from build123d import *

# Parameters (mm, degrees)
SKETCH_3_R               = 3
EXTRUDE_6_DEPTH          = 0.001
EXTRUDE_6_2_DEPTH        = 0.001
EXTRUDE_6_3_DEPTH        = 0.001
EXTRUDE_6_4_DEPTH        = 0.001
SKETCH_11_R              = 2.25
CUT_EXTRUDE_2_DEPTH      = 1
CUT_EXTRUDE_2_DEPTH_BACK = 1.001
EXTRUDE_7_DEPTH          = 3
SKETCH_14_R              = 2.25
SKETCH_14_R_2            = 10
CUT_EXTRUDE_3_DEPTH      = 3
SKETCH_15_R              = 10
SKETCH_15_R_2            = 2.5
CUT_EXTRUDE_4_DEPTH      = 3
SKETCH_16_R              = 1.5
CUT_EXTRUDE_5_DEPTH      = 10
SKETCH_17_R              = 9.5
SKETCH_17_R_2            = 7.5
EXTRUDE_8_DEPTH          = 4.9
FILLET_1_R               = 10


with BuildPart() as part:
    # Sketch 3 → Extrude 6 (new body)
    with BuildSketch(Plane.XY):
        with Locations((60.266478541, 16.532501821)):
            Circle(SKETCH_3_R)
    extrude(amount=EXTRUDE_6_DEPTH)


with BuildPart() as body_2:
    # Sketch 3 → Extrude 6 2 (new body)
    with BuildSketch(Plane.XY):
        with Locations((60.266478541, 6.532501821)):
            Circle(SKETCH_3_R)
    extrude(amount=EXTRUDE_6_2_DEPTH)


with BuildPart() as body_3:
    # Sketch 3 → Extrude 6 3 (new body)
    with BuildSketch(Plane.XY):
        with Locations((10.766478541, 6.532501821)):
            Circle(SKETCH_3_R)
    extrude(amount=EXTRUDE_6_3_DEPTH)


with BuildPart() as body_4:
    # Sketch 3 → Extrude 6 4 (new body)
    with BuildSketch(Plane.XY):
        with Locations((10.766478541, 16.532501821)):
            Circle(SKETCH_3_R)
    extrude(amount=EXTRUDE_6_4_DEPTH)


with BuildPart() as cut_extrude_2_tool:
    # Sketch 11 → Cut-Extrude 2 (new body, two sides)
    with BuildSketch(Plane.XY.offset(0.001)) as cut_extrude_2_sk:
        with Locations((10.766478541, 16.532501821)):
            Circle(SKETCH_11_R)
        with Locations((10.766478541, 6.532501821)):
            Circle(SKETCH_11_R)
        with Locations((60.266478541, 16.532501821)):
            Circle(SKETCH_11_R)
        with Locations((60.266478541, 6.532501821)):
            Circle(SKETCH_11_R)
    extrude(amount=CUT_EXTRUDE_2_DEPTH)
    extrude(cut_extrude_2_sk.sketch, amount=-CUT_EXTRUDE_2_DEPTH_BACK)


with BuildPart() as part_1:
    add(part.part)

    # Cut-Extrude 2: cut by cut_extrude_2_tool
    add(cut_extrude_2_tool.part, mode=Mode.SUBTRACT)



with BuildPart() as body_2_1:
    add(body_2.part)

    # Cut-Extrude 2: cut by cut_extrude_2_tool
    add(cut_extrude_2_tool.part, mode=Mode.SUBTRACT)


with BuildPart() as body_3_1:
    add(body_3.part)

    # Cut-Extrude 2: cut by cut_extrude_2_tool
    add(cut_extrude_2_tool.part, mode=Mode.SUBTRACT)


with BuildPart() as body_4_1:
    add(body_4.part)

    # Cut-Extrude 2: cut by cut_extrude_2_tool
    add(cut_extrude_2_tool.part, mode=Mode.SUBTRACT)


with BuildPart() as part_2:
    add(part_1.part)

    add(body_2_1.part)  # Extrude 7 merges body 2

    add(body_3_1.part)  # Extrude 7 merges body 3

    add(body_4_1.part)  # Extrude 7 merges body 4
    # Sketch 12 → Extrude 7 (add)
    with BuildSketch(Plane.XY.offset(0.001)):
        Polygon((5.516478541, 26.532501821), (65.516478541, 26.532501821), (65.516478541, -38.467498179), (5.516478541, -38.467498179), (5.516478541, 1.532501821), align=None)
    extrude(amount=EXTRUDE_7_DEPTH)

    # Sketch 14 → Cut-Extrude 3 (cut)
    with BuildSketch(Plane(origin=(0, 0, 0.001), x_dir=(-1, 0, 0), z_dir=(0, 0, -1))):
        with Locations((-60.266478541, 6.532501821)):
            Circle(SKETCH_14_R)
        with Locations((-60.266478541, 16.532501821)):
            Circle(SKETCH_14_R)
        with Locations((-10.766478541, 6.532501821)):
            Circle(SKETCH_14_R)
        with Locations((-10.766478541, 16.532501821)):
            Circle(SKETCH_14_R)
        with Locations((-45.516478541, 11.532501821)):
            Circle(SKETCH_14_R_2)
    extrude(amount=-CUT_EXTRUDE_3_DEPTH, mode=Mode.SUBTRACT)

    # Sketch 15 → Cut-Extrude 4 (cut)
    with BuildSketch(Plane(origin=(0, 0, 0.001), x_dir=(-1, 0, 0), z_dir=(0, 0, -1))):
        with Locations((-45.516478541, 11.532501821)):
            Circle(SKETCH_15_R)
        with Locations((-45.516478541, -28.467498179)):
            Circle(SKETCH_15_R_2)
    extrude(amount=-CUT_EXTRUDE_4_DEPTH, mode=Mode.SUBTRACT)

    # Sketch 16 → Cut-Extrude 5 (cut)
    with BuildSketch(Plane.XY.offset(3.001)):
        with Locations((10.516478541, -9.467498179)):
            Circle(SKETCH_16_R)
        with Locations((22.516478541, -9.467498179)):
            Circle(SKETCH_16_R)
    extrude(amount=-CUT_EXTRUDE_5_DEPTH, mode=Mode.SUBTRACT)

    # Sketch 17 → Extrude 8 (add)
    with BuildSketch(Plane.XY.offset(3.001)):
        with Locations((45.516478541, -28.467498179)):
            Circle(SKETCH_17_R)
        with Locations((45.516478541, -28.467498179)):
            Circle(SKETCH_17_R_2, mode=Mode.SUBTRACT)
    extrude(amount=-EXTRUDE_8_DEPTH)

    # Fillet 1
    fillet_1_edges = [part_2.edges().sort_by_distance(p)[0] for p in [
        (5.516478541, 26.532501821, 1.501),
        (5.516478541, -38.467498179, 1.501),
        (65.516478541, -38.467498179, 1.501),
        (65.516478541, 26.532501821, 1.501),
    ]]
    fillet(fillet_1_edges, radius=FILLET_1_R)


solid = part_2.part
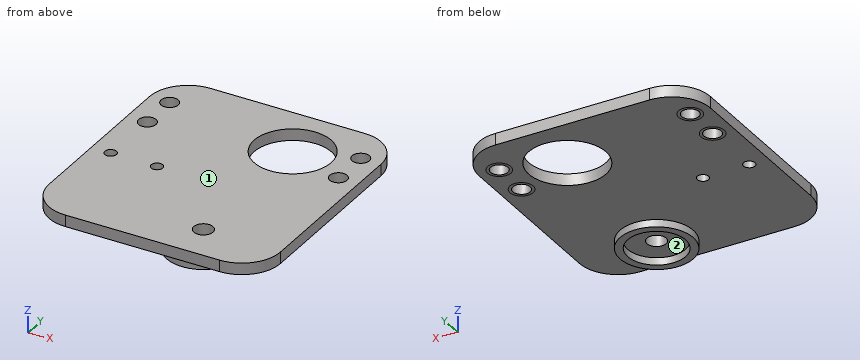
Source: CAD feature listing. Evaluate the final solid. Frame: model axes, mm. Face numbers are marked on the shaded views. Coordinates: 2 decimals unless noted, no trailing zeros. Loops run counter-clockwise (first coordinate to the right, second up) from the corner with the lowest first, then second, coordinate; pieces in that order, holes last. Notation, with made-up numbers: (-3, 59.5) - (8, 59.5) arc R17 cw to (8, 79.5) - close; hole circle Ø11 at (63.25, 21.25). An arc over 180 degrees is marked (long way). One line per item, written item: value. Start each with the question number.
1. Mould query, pull axis Y, two halves, no side actions, for the marked faces 1 and 2. Classes: pulls with the +Y half, pulls with the -Y half, needs draft (parallel to the pull), parting line crosses it, or undercut.
2. Section B-B (y = -27.5). Return the cut outline in (x, z), and give its area (3 significant figures).
3. Contact query for flat-ended pins moving along their axis: P1, Ø5, axis at x = 59, y = 8, coming from the -Z side; P2, Ø2.5, axis at x = 10.77, y = 6.53, coming from the -Z side. Output: stop coordinate, or through.
4. Ray query, L1, parallel to X at y = -9.5, z = 0.6; L2, parallel to X at y = 7.5, z = 1.2; L3, parallel to X at y = 18, z = 2.1. Return the intervals inside material, ascending.
5. Section A-A (x = 50.5). Return the cut outline in (y, z).
6. Section C-C (y = 8). State how many separate pieces and enclosed holes the cut face has, and give its area (3 significant figures).
Verdict:
1. face 1: needs draft
1. face 2: undercut
2. outline: (5.52, 0) - (36.07, 0) - (36.07, -1.9) - (38.08, -1.9) - (38.08, 0) - (43.21, 0) - (43.21, 3) - (5.52, 3) - close; (47.82, 0) - (52.95, 0) - (52.95, -1.9) - (54.97, -1.9) - (54.97, 0) - (65.52, 0) - (65.52, 3) - (47.82, 3) - close
2. area: 174 mm2
3. P1: stops at z = 0
3. P2: passes through
4. L1: x = 5.52 to 9.02, 12.02 to 21.02, 24.02 to 65.52
4. L2: x = 5.52 to 8.74, 12.8 to 36.37, 54.67 to 58.24, 62.3 to 65.52
4. L3: x = 5.62 to 9.06, 12.47 to 37.89, 53.14 to 58.56, 61.97 to 65.41
5. outline: (-38.47, 0) - (-36.56, 0) - (-36.56, -1.9) - (-34.07, -1.9) - (-34.07, 0) - (-22.86, 0) - (-22.86, -1.9) - (-20.38, -1.9) - (-20.38, 0) - (2.86, 0) - (2.86, 3) - (-38.47, 3) - close; (20.2, 0) - (26.53, 0) - (26.53, 3) - (20.2, 3) - close
6. separate pieces: 4
6. enclosed holes: 0
6. area: 103 mm2
